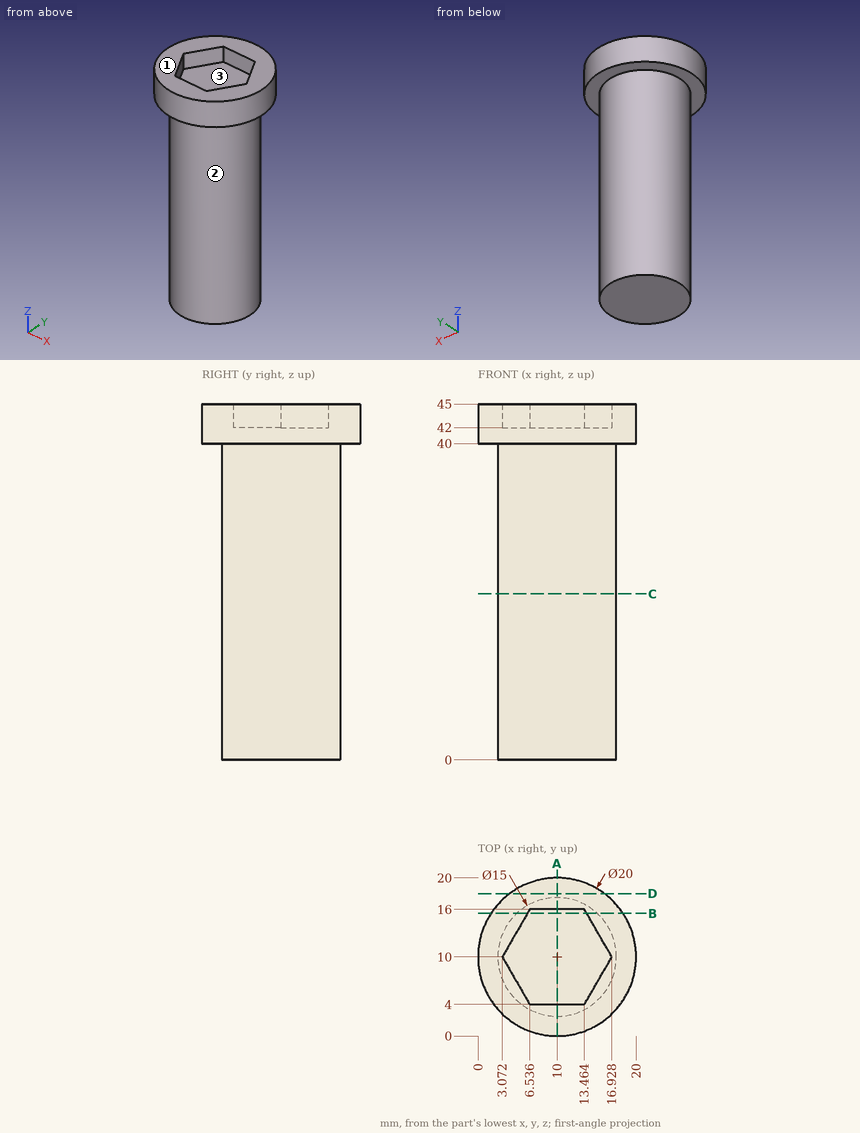
Check sheet for the drawn part. Datum: minimum x, y, z corner. Units: mm. Coordinates: 2 decimals unless noted, no trailing zeros. Loops run counter-clockwise (first coordinate to the right, second up) from the corner with the lowest first, then second, coordinate; pieces in that order, holes last. Notation, with made-up numbers: (-22, -2.5) -> (37, -2.5) arc R19 cw to (37, 17.5) -> close; hole circle Ø10 at (82.5, 62.5). An arc over 180 degrees is marked (long way). Answer in a Markdown table with one row per item.
1) Draft check along X on the marked faces 1, 2 and 3. Enter one of: released by +X, released by -X, zero draft, split by the parting line, or undercut.
The answers:
| item | result |
|---|---|
| face 1 | zero draft |
| face 2 | split by the parting line |
| face 3 | undercut |
2) Scan lines: line 1 along Y through (x, z) = (18, 40.5); line 2 along Z through (x, y) = (4.75, 7.5); line 3 along Z through (x, y) = (6, 17.75). Record each from-to range of solid material in increasing order. Write a range as from..to.
The answers:
| item | result |
|---|---|
| line 1 | y = 4..16 |
| line 2 | z = 0..42 |
| line 3 | z = 40..45 |
3) Section check A-A (x = 10). Record the cut outline in (y, z).
The answers:
| item | result |
|---|---|
| outline | (0, 40) -> (2.5, 40) -> (2.5, 0) -> (17.5, 0) -> (17.5, 40) -> (20, 40) -> (20, 45) -> (16, 45) -> (16, 42) -> (4, 42) -> (4, 45) -> (0, 45) -> close |
4) Depth check by flat-ended pin: P1, Ø4, axis at y = 15, z = 35.5, coming from the -X side; P2, Ø4, axis at y = 5.5, z = 36.5, coming from the -X side; P3, Ø2.5, axis at x = 11.5, z = 43.5, coming from the -Y side; P4, Ø10, axis at x = 7, y = 5.5, coming from the -Z side. Enter the tip coordinate at first touch or a pass-through.
The answers:
| item | result |
|---|---|
| P1 | stops at x = 3.13 |
| P2 | stops at x = 2.93 |
| P3 | stops at y = 0 |
| P4 | stops at z = 0 |
5) Section check B-B (y = 15.5). Record the cut outline in (x, z).
The answers:
| item | result |
|---|---|
| outline | (1.65, 40) -> (4.9, 40) -> (4.9, 0) -> (15.1, 0) -> (15.1, 40) -> (18.35, 40) -> (18.35, 45) -> (13.75, 45) -> (13.75, 42) -> (6.25, 42) -> (6.25, 45) -> (1.65, 45) -> close |
6) Section check D-D (y = 18). Record the cut outline in (x, z).
The answers:
| item | result |
|---|---|
| outline | (4, 40) -> (16, 40) -> (16, 45) -> (4, 45) -> close |
7) Section check C-C (z = 21). Record the cut outline in (x, y).
The answers:
| item | result |
|---|---|
| outline | circle Ø15 at (10, 10) |
